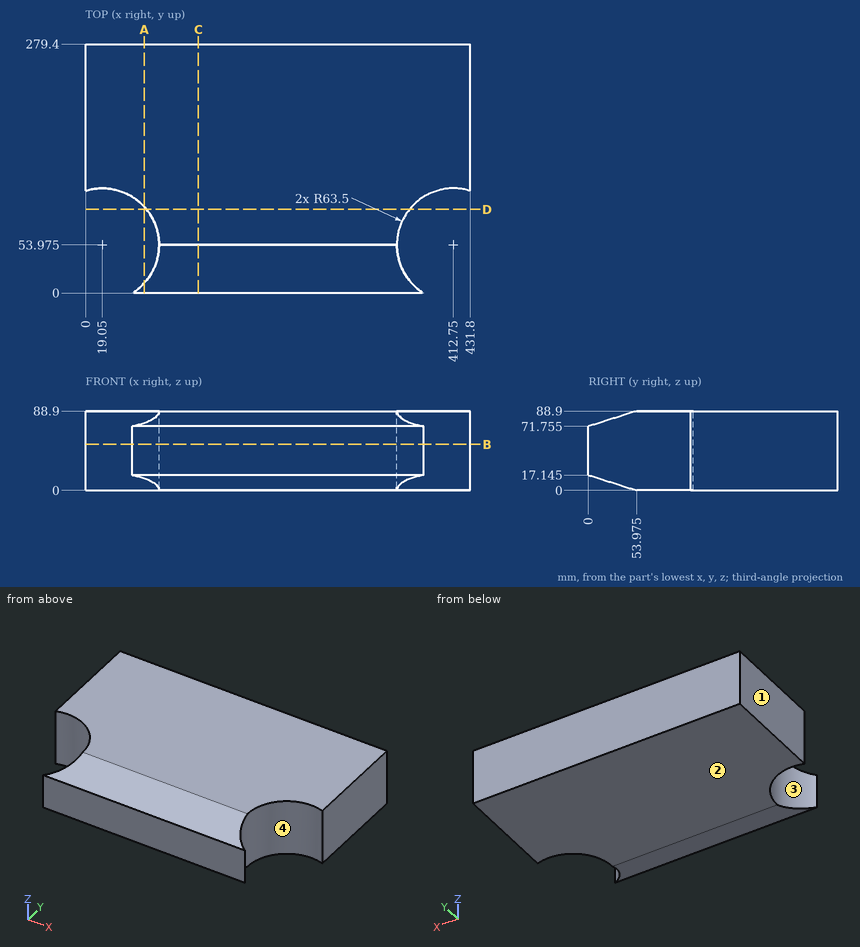
Could you check a few things on this drawing? It's one solid part, dimensions in mm from its lowest x, y, z. Coordinates: 2 decimals unless noted, no trailing zeros. Write each loop counter-clockwise with the first axis right and the second up, starting at its lowest first coordinate (ties: lowest second). Pieces come first, ordered by that corner, then holes. Notation, with made-up numbers: M -14.75,77 L 41.25,77 A21 cw 41.25,115 Z; hole C 58,-13.5 d6. An arc over 180 degrees is marked long. Answer as CSV lines item,"result". Start each with the question number.
Q1. Suppose I cut it at D-D, the plane y = 94. List the corners of the cut face in (x, z) for me, then the cut area to 3 significant figures.
Q2. Suppose I cut it at B-B, the plane z = 51.5. List the corners of the cut face in (x, y) for me (3 decimals).
Q3. Will these pins go through, and if not, where does the flat tip stop? pin 1 Ø10 at (y, z) = (46, 62) entering from +X; pin 2 Ø2 at (y, z) = (57.5, 49.5) entering from +X.
Q4. I need wall thicknesses on probe 1 along Y at (x, z) = (371, 76.5); probe 2 along Y at (x, z) = (56, 8); probe 3 along X at (y, z) = (107.5, 48.5). Which ranges of each line are inside material? Lowest first, please. Write a range as [from, to].
Q5. If we mould it in two halves opening along X, with no side actions, what happens to the marked faces 1, 2, 3 and 4? For each: pulls with the +X half, pulls with the -X half, needs draft (parallel to the pull), parting line crosses it, or undercut.
Q6. Suppose I cut it at A-A, the plane x = 66. List the corners of the cut face in (y, z) for me (1 decimal), then the cut area to 3 significant figures.
Q7. Suppose I cut it at C-C, the plane x = 126.5. List the corners of the cut face in (y, z) for me (3 decimals), then the cut area to 3 significant figures.
Entries:
1,outline,"M 68.35,0 L 363.45,0 L 363.45,88.9 L 68.35,88.9 Z"
1,area,"26,200 mm²"
2,outline,"M 0,114.55 A63.5 cw 52.501,0 L 379.299,0 A63.5 cw 431.8,114.55 L 431.8,279.4 L 0,279.4 Z"
3,pin 1,"stops at x = 350.59"
3,pin 2,"stops at x = 349.41"
4,probe 1,"y = [101.82, 279.4]"
4,probe 2,"y = [105.62, 279.4]"
4,probe 3,"x = [53.22, 378.58]"
5,face 1,"pulls with the -X half"
5,face 2,"needs draft"
5,face 3,"undercut"
5,face 4,"undercut"
6,outline,"M 0,17.1 L 11.2,13.6 L 11.2,75.3 L 0,71.8 Z; M 96.7,0 L 279.4,0 L 279.4,88.9 L 96.7,88.9 Z"
6,area,"16,900 mm²"
7,outline,"M 0,17.145 L 53.975,0 L 279.4,0 L 279.4,88.9 L 53.975,88.9 L 0,71.755 Z"
7,area,"23,900 mm²"
